Autodesk Inventor part; units mm, degrees
ref_plane "YZ Plane" through (0, 0, 0) normal (1, 0, 0) x (0, 1, 0)
ref_plane "XZ Plane" through (0, 0, 0) normal (0, 1, 0) x (-1, 0, 0)
ref_plane "XY Plane" through (0, 0, 0) normal (0, 0, 1) x (1, 0, 0)
sketch "Boceto1" plane through (0, 0, 0) normal (0, 0, 1) x (1, 0, 0)
  line L0 (0, 0) -> (0, 19.566)
  line L1 (2, 65) -> (2, 21)
  line L2 (2, 21) -> (0, 19.566)
  line L3 (2, 65) -> (14.5, 65)
  line L4 (29, 0) -> (29, 19.566)
  line L5 (27, 65) -> (27, 21)
  line L6 (27, 21) -> (29, 19.566)
  line L7 (27, 65) -> (14.5, 65)
  line L8 (0, 0) -> (29, 0)
extrude "Extrusión1" add sketch "Boceto1" along normal blind 7
sketch "Boceto2" plane through (0, 0, 7) normal (0, 0, 1) x (1, 0, 0)
  line L0 (27, 65) -> (27, 21)
  line L1 (2, 65) -> (27, 65)
  line L2 (2, 21) -> (2, 65)
  line L3 (2, 65) -> (5, 65)
  line L4 (2, 65) -> (2, 26)
  line L5 (5, 26) -> (5, 65)
  line L6 (27, 65) -> (24, 65)
  line L7 (24, 65) -> (24, 41)
  line L8 (27, 65) -> (27, 26)
  line L9 (5, 26) -> (2, 26)
  line L10 (24, 26) -> (27, 26)
  line L11 (24.1227, 26) -> (22, 26)
  line L12 (22, 26) -> (22, 41)
  line L13 (22, 41) -> (24, 41)
  dimension "d7" = 15
extrude "Extrusión2" add sketch "Boceto2" along normal blind 9
sketch "Boceto3" plane through (0, 0, 7) normal (0, 0, 1) x (1, 0, 0)
  line L0 (5, 65) -> (24, 65)
  line L1 (29, 0) -> (0, 0)
  line L2 (22, 41) -> (24, 41)
  line L3 (2, 0.5) -> (2, 21)
  line L4 (2, 21) -> (5, 21)
  line L5 (5, 21) -> (5, 0.5)
  line L6 (5, 0.5) -> (2, 0.5)
  line L7 (27, 0.5) -> (27, 21)
  line L8 (27, 21) -> (24, 21)
  line L9 (24, 21) -> (24, 0.5)
  line L10 (24, 0.5) -> (27, 0.5)
  dimension "d9" = 20.5
extrude "Extrusión3" add sketch "Boceto3" along normal blind 5
sketch "Boceto4" plane through (0, 0, 7) normal (0, 0, 1) x (1, 0, 0)
  line L0 (29, 0) -> (0, 0)
  line L1 (7, 10) -> (13, 10)
  line L2 (13, 10) -> (13, 27)
  line L3 (13, 27) -> (7, 27)
  line L4 (7, 27) -> (7, 10)
extrude "Extrusión4" add sketch "Boceto4" along normal blind 4
properties part number "fio"
Input: part model. Units: mm. Frame: model coordinates. A direction names the side the tool comes from. Give positions to 0.01 mm unless a question says otherwise; leave off trailing zeros. Order: outer loops, then holes, each group sorted by start corner. A loop starts at its lowest first (then second) coordinate and runs counter-clockwise, first axis right, second up. Notation, with made-up numbers: (-26.75, 58) - (8.25, 58) arc R25 cw to (8.25, 72) - close; hole circle Ø2 at (5, -5). An arc over 180 degrees is marked (long way). Write each question's results on one line, items separated by ' | '.
Item 1: Section C-C (z = 8.75). Return loops of the section in (x, y), and give its area (3 significant figures).
A:
outline: (2, 0.5) - (5, 0.5) - (5, 21) - (2, 21) - close; (2, 26) - (5, 26) - (5, 65) - (2, 65) - close; (7, 10) - (13, 10) - (13, 27) - (7, 27) - close; (22, 26) - (27, 26) - (27, 65) - (24, 65) - (24, 41) - (22, 41) - close; (24, 0.5) - (27, 0.5) - (27, 21) - (24, 21) - close | area: 489 mm^2
Item 2: Section B-B (y = 5). Return loops of the section in (x, z).
A:
outline: (0, 0) - (29, 0) - (29, 7) - (27, 7) - (27, 12) - (24, 12) - (24, 7) - (5, 7) - (5, 12) - (2, 12) - (2, 7) - (0, 7) - close
Item 3: Section A-A (z = 13.75). Return loops of the section in (x, y), and give its area (3 significant figures).
A:
outline: (2, 26) - (5, 26) - (5, 65) - (2, 65) - close; (22, 26) - (27, 26) - (27, 65) - (24, 65) - (24, 41) - (22, 41) - close | area: 264 mm^2
Item 4: Access query for faces 4 (the flat face through (25, 11, 12)), 5 (the flat face through (2, 11, 9)), 6 (the flat face through (24, 11, 9)), 7 (the flat face through (27, 11, 9)), 8 (the flat face through (10, 27, 9)). Directions: +Z, -Z, +X, -X, +Y, -Y. A direction counts if a zero-diameter tool reaches every point of the face in a straight line with its end or side. Return the directions, or none.
A:
face 4: +Z, +X, -X, -Y | face 5: +Z, -X, +Y, -Y | face 6: +Z, -Y | face 7: +Z, +X, +Y, -Y | face 8: +Z, +Y
Item 5: Material intervals for line 1 along X through (y, z) = (45.5, 14); line 2 along X through (y, z) = (30, 9.75); line 3 along Z through (x, y) = (13, 6.5), sorted ascending.
A:
line 1: x = 2 to 5, 24 to 27 | line 2: x = 2 to 5, 22 to 27 | line 3: z = 0 to 7
Item 6: Draft query along Y for faces 1 (the flat face through (27, 43, 8)), 2 (the flat face through (26, 21, 9)), 3 (the flat face through (10, 10, 9)). Return one class per face: released by +Y, released by -Y, zero draft, split by the parting line, or undercut.
A:
face 1: zero draft | face 2: undercut | face 3: released by -Y
Item 7: Section D-D (x = 10.75). Return loops of the section in (y, z), and give its area (3 significant figures).
A:
outline: (0, 0) - (65, 0) - (65, 7) - (27, 7) - (27, 11) - (10, 11) - (10, 7) - (0, 7) - close | area: 523 mm^2
Item 8: Contact query for flat-ended pins moving along their axis: pin 1 Ø5 at (y, z) = (44.5, 9.5) entering from +X; pin 2 Ø1.2 at (x, z) = (9.5, 8.5) entering from +Y; pin 3 Ø5 at (y, z) = (35.5, 11.5) entering from -X. Output: stop coordinate, or through.
A:
pin 1: stops at x = 27 | pin 2: stops at y = 27 | pin 3: stops at x = 2
